Can you work these out from the model? Positions are in its coordinate system, mm. Coordinates: 2 decimals unless noted, no trailing zeros. Write each loop counter-clockwise with the first axis right and the second up, starting at its lowest first coordinate (ties: lowest second). Pieces come first, ordered by that corner, then holes. Notation, with made-up numbers: (2.25, 65) -> (34.25, 65) arc R31 cw to (34.25, 98) -> close; hole circle Ø11 at (65.25, 5). An arc over 180 degrees is marked (long way). Answer as CSV lines item,"result". Start each with the question number.
```python
from build123d import *

# Parameters (mm, degrees)
SKETCH1_W                  = 180
SKETCH1_H                  = 130
BOSS_EXTRUDE1_DEPTH        = 3
FILLET1_R                  = 40
FILLET2_R                  = 40
F_10_0_10_DIAMETER_HOLE1_D = 10
F_3_2_3_2_DIAMETER_HOLE1_D = 3.2


with BuildPart() as part:
    # Sketch1 → Boss-Extrude1 (new body)
    with BuildSketch(Plane(origin=(0, 0, 0), x_dir=(1, 0, 0), z_dir=(0, 1, 0))):
        Rectangle(SKETCH1_W, SKETCH1_H)
    extrude(amount=BOSS_EXTRUDE1_DEPTH)

    # Fillet1
    fillet1_edges = [part.edges().sort_by_distance(p)[0] for p in [
        (-90, 1.5, 65),
        (-90, 1.5, -65),
    ]]
    fillet(fillet1_edges, radius=FILLET1_R)

    # Fillet2
    fillet2_edges = [part.edges().sort_by_distance(p)[0] for p in [
        (90, 1.5, 65),
        (90, 1.5, -65),
    ]]
    fillet(fillet2_edges, radius=FILLET2_R)

    # Ø10.0 (10) Diameter Hole1 (through all)
    with Locations(Plane(origin=(0, 3, 0), x_dir=(1, 0, 0), z_dir=(0, 1, 0))):
        with Locations((45, 0), (-45, 0)):
            Hole(F_10_0_10_DIAMETER_HOLE1_D / 2)

    # Ø3.2 (3.2) Diameter Hole1 (through all)
    with Locations(Plane(origin=(-70, 3, -45), x_dir=(0, 0, 1), z_dir=(0, 1, 0))):
        with Locations((0, 0), (0, 70), (0, 140), (90, 0), (90, 70), (90, 140)):
            Hole(F_3_2_3_2_DIAMETER_HOLE1_D / 2)


solid = part.part
```
Q1. If we mould it in two halves opening along X, with no side actions, what happens to faces 1 (the face through (-78.594, 1.521, -52.972)), 2 (the face through (-40, 1, 0)), 3 (the face through (-1, 3, -1))? For each: released by +X, released by -X, zero draft, split by the parting line, or undercut.
Q2. Imagine slicing it at D-D (z = 53.5). Write out the boundary of the cut face in (x, y), then the cut area to 3 significant figures.
Q3. Imagine slicing it at A-A (x = -45). Write out the boundary of the cut face in (y, z), then the cut area to 3 significant figures.
Q4. For pin 1 (2.5 mm diameter, centred on x = 0, z = 45, fed in from -Y); pin 2 (1.5 mm diameter, centred on y = 1.5, z = 49, fed in from -X); pin 3 (1 mm diameter, centred on y = 1, z = 27, fed in from +X), each with a flat end and sliding along its axis, tell me the tip position at first contact or that it passes through.
Q5. I need wall thicknesses on L1, parallel to X at y = 0.6, z = 0.5; L2, parallel to Z at x = -45, y = 0.8; L3, parallel to X at y = 0.95, z = -45. Which ranges of each line are inside material? Lowest first, please.
Q6. Imagine slicing it at C-C (z = 0). Write out the boundary of the cut face in (x, y).
Q7. Imagine slicing it at B-B (y = 2.4). State how many separate pieces and enclosed holes the cut face has, then the cut area to 3 significant figures.
Entries:
1,face 1,"released by -X"
1,face 2,"undercut"
1,face 3,"zero draft"
2,outline,"(-78.07, 0) -> (78.07, 0) -> (78.07, 3) -> (-78.07, 3) -> close"
2,area,"468 mm2"
3,outline,"(0, -65) -> (3, -65) -> (3, -5) -> (0, -5) -> close; (0, 5) -> (3, 5) -> (3, 65) -> (0, 65) -> close"
3,area,"360 mm2"
4,pin 1,"through"
4,pin 2,"x = -82.55"
4,pin 3,"x = 89.97"
5,L1,"-90 to -49.97, -40.03 to 40.03, 49.97 to 90"
5,L2,"-65 to -5, 5 to 65"
5,L3,"-84.64 to -71.6, -68.4 to -1.6, 1.6 to 68.4, 71.6 to 84.64"
6,outline,"(-90, 0) -> (-50, 0) -> (-50, 3) -> (-90, 3) -> close; (-40, 0) -> (40, 0) -> (40, 3) -> (-40, 3) -> close; (50, 0) -> (90, 0) -> (90, 3) -> (50, 3) -> close"
7,separate pieces,"1"
7,enclosed holes,"8"
7,area,"21,800 mm2"
